from build123d import *

# Parameters (mm, degrees)
SKETCH_R     = 5
SKETCH_R_2   = 2.5
PAD_DEPTH    = 5
POCKET_DEPTH = 1
FILLET_R     = 1


with BuildPart() as part:
    # Sketch → Pad (new body)
    with BuildSketch(Plane.XY):
        with BuildLine():
            Line((-21, 22), (21, 22))
            ThreePointArc((27.5, 15.5), (25.596194, 20.096194), (21, 22))
            Line((27.5, 15.5), (27.5, -15.5))
            ThreePointArc((21, -22), (25.596194, -20.096194), (27.5, -15.5))
            Line((21, -22), (-21, -22))
            ThreePointArc((-27.5, -15.5), (-25.596194, -20.096194), (-21, -22))
            Line((-27.5, -15.5), (-27.5, 15.5))
            ThreePointArc((-21, 22), (-25.596194, 20.096194), (-27.5, 15.5))
        make_face()
        Circle(SKETCH_R, mode=Mode.SUBTRACT)
        with Locations((-21, 15.5)):
            Circle(SKETCH_R_2, mode=Mode.SUBTRACT)
        with Locations((21, 15.5)):
            Circle(SKETCH_R_2, mode=Mode.SUBTRACT)
        with Locations((21, -15.5)):
            Circle(SKETCH_R_2, mode=Mode.SUBTRACT)
        with Locations((-21, -15.5)):
            Circle(SKETCH_R_2, mode=Mode.SUBTRACT)
    extrude(amount=PAD_DEPTH)

    # Sketch001 (on Face15 of Pad) → Pocket (cut)
    with BuildSketch(Plane.XY.offset(5)):
        Polygon((8.5, 4.907477), (0, 9.814955), (-8.5, 4.907477), (-8.5, -4.907477), (0, -9.814955), (8.5, -4.907477), align=None)
    extrude(amount=-POCKET_DEPTH, mode=Mode.SUBTRACT)

    # Fillet
    fillet_edges = [part.edges().sort_by_distance(p)[0] for p in [
        (25.596194, -20.096194, 0),
        (0, -22, 0),
        (27.5, 0, 0),
        (25.596194, 20.096194, 0),
        (0, 22, 0),
        (-25.596194, 20.096194, 0),
        (-27.5, 0, 0),
        (-25.596194, -20.096194, 0),
    ]]
    fillet(fillet_edges, radius=FILLET_R)


solid = part.part
Verification items for the finished model (mm, model axes). A direction names the side the tool comes from. Coordinates: 2 decimals unless noted, no trailing zeros. Order: outer loops, then holes, each group sorted by start corner. A loop starts at its lowest first (then second) coordinate and runs counter-clockwise, first axis right, second up. Notation, with made-up numbers: M 43.5,-10 L 65.5,-10 A23 ccw 65.5,-2 Z; hole C -7.75,-33 d2. An arc over 180 degrees is marked long. Write each question's results on one line, items separated by ' | '.
1) Scan lines: line 1 along Y through (x, z) = (-21, 3.5); line 2 along Y through (x, z) = (23, 0.7); line 3 along Y through (x, z) = (0, 3.1). Record each from-to range of solid material in increasing order. Write a range as [from, to].
Solved:
line 1: y = [-22, -18], [-13, 13], [18, 22] | line 2: y = [-21.64, -17], [-14, 14], [17, 21.64] | line 3: y = [-22, -5], [5, 22]
2) Section check C-C on y = -16.5. Give the number of separate pieces and of enclosed holes in the cut face, plus the area to 3 significant figures.
Solved:
separate pieces: 3 | enclosed holes: 0 | area: 228 mm²
3) Access from +Z, -Z, +X, -X, +Y, -Y to the whole of each face (thin tool, end or side, straight path). Record for faces 5 (the face through (27.5, 0, 3)), 6 (the face through (4.19, -7.396, 4.507)).
Solved:
face 5: +Z, -Z, +X, +Y, -Y | face 6: +Z
4) Section check A-A on z = 2.5. Record the cut outline in (x, y), plus the area to 3 significant figures.
Solved:
outline: M -27.5,-15.5 A6.5 ccw -21,-22 L 21,-22 A6.5 ccw 27.5,-15.5 L 27.5,15.5 A6.5 ccw 21,22 L -21,22 A6.5 ccw -27.5,15.5 Z; hole C -21,-15.5 d5; hole C -21,15.5 d5; hole C 0,0 d10; hole C 21,-15.5 d5; hole C 21,15.5 d5 | area: 2,230 mm²
5) Section check B-B on y = 0. Record the cut outline in (x, z), plus the area to 3 significant figures.
Solved:
outline: M -27.5,1 A1 ccw -26.5,0 L -5,0 L -5,4 L -8.5,4 L -8.5,5 L -27.5,5 Z; M 5,0 L 26.5,0 A1 ccw 27.5,1 L 27.5,5 L 8.5,5 L 8.5,4 L 5,4 Z | area: 218 mm²
6) Gauge pin test, flat ends, axial feed: pin 1 Ø8 at (x, y) = (-21, -15.5) entering from +Z; pin 2 Ø3 at (x, y) = (-21, 15.5) entering from -Z; pin 3 Ø6 at (x, y) = (3, -1) entering from +Z. Record the tip position at first contact, or that the pin passes through.
Solved:
pin 1: stops at z = 5 | pin 2: passes through | pin 3: stops at z = 4
7) Release check for a two-part mould opening along X. For faces 1 (the face through (18.5, -15.4, 2.5)), 2 (the face through (25.545, -20.146, 2.972)), 3 (the face through (-25.646, -20.045, 2.972)), 4 (the face through (0, -22, 3)) record: pulls with the +X half, pulls with the -X half, needs draft (parallel to the pull), parting line crosses it, or undercut.
Solved:
face 1: undercut | face 2: pulls with the +X half | face 3: pulls with the -X half | face 4: needs draft
